Can you work these out from the model? Positions are in its coordinate system, mm. A direction names the side the tool comes from. Give positions to 0.01 mm unless a question says otherwise; leave off trailing zeros. Loops run counter-clockwise (first coordinate to the right, second up) from the corner with the lowest first, then second, coordinate; pieces in that order, holes last. Notation, with made-up numbers: (32.25, 85.25) -> (90.25, 85.25) arc R11 ccw to (90.25, 103.25) -> close; hole circle Ø7 at (34, -32). An arc over 180 degrees is marked (long way). Return JSON: item names as keys, results as strings. Group by question number.
Q1. Will these pins go through, and if not, where does the flat tip stop? pin 1 (12 mm diameter, centred on x = 30.5, y = 23, fed in from -Z); pin 2 (8 mm diameter, centred on y = 22.5, z = -41.5, fed in from -X); pin 3 (3 mm diameter, centred on y = 55, z = -5, fed in from -X) (1 decimal); pin 4 (2 mm diameter, centred on y = 52, z = -27.5, fed in from +X).
Q2. Which directions (+Z, -Z, +X, -X, +Y, -Y) give clear straight access to the entire face, cutting with the end or side of a thin tool? Please do faces 1 (the cylindrical face through (28, 38, -28)), 2 (the cylindrical face through (40, 12, -6)), 3 (the flat face through (20, 53, -7)).
Q3. I need wall thicknesses on line 1 along Z through (x, y) = (15.75, 55); line 2 along Y through (x, z) = (67, -55); line 3 along Z through (x, y) = (71, 3). Which ranges of each line are inside material? Lowest first, please. Write a range as [from, to].
Q4. Suppose I cut it at A-A, the plane z = -15.5. Please give me the cut outline in (x, y), and give its area (3 significant figures).
Q5. Suppose I cut it at B-B, the plane y = 9.5. Please give me the cut outline in (x, z), and give its area (3 significant figures).
Q6. Suppose I cut it at C-C, the plane x = 55. Please give me the cut outline in (y, z).
Q7. Thinking about a two-plate mould opening in Z: for faces 4 (the flat face through (60, 7, -53)), 5 (the cylindrical face through (10, 59, -58)), 6 (the flat face through (98, 35, -32.5)), which applies, pulls with the +Z half, pulls with the -Z half, needs draft (parallel to the pull), parting line crosses it, or undercut?
```python
from build123d import *

# Parameters (mm, degrees)
SKETCH_1_W           = 60
SKETCH_1_H           = 60
EXTRUDE_1_DEPTH      = 20
SKETCH_2_R           = 30
EXTRUDE_2_DEPTH      = 40
SKETCH_3_W           = 60
SKETCH_3_H           = 60
EXTRUDE_3_DEPTH      = 12
SKETCH_4_R           = 22
EXTRUDE_4_DEPTH      = 10
SKETCH_5_R           = 7
EXTRUDE_5_DEPTH      = 22
SKETCH_6_R           = 2.5
CUT_EXTRUDE_1_DEPTH  = 135.223693885
SKETCH_7_R           = 25
CUT_EXTRUDE_2_DEPTH  = 5
SKETCH_8_R           = 7
CUT_EXTRUDE_3_DEPTH  = 25
CUT_EXTRUDE_START    = -15
CUT_EXTRUDE_5_DEPTH  = 15
FILLET_1_R           = 2.5
SKETCH_11_R          = 8
EXTRUDE_6_DEPTH      = 2
M5X0_751_D           = 4.2
M5X0_751_DEPTH       = 14
M5X0_751_CSINK_D     = 6
M5X0_751_CSINK_ANGLE = 90
M5X0_751_TIP         = 1.2618073
FILLET_2_R           = 5
SKETCH_15_W          = 5
SKETCH_15_H          = 2.461651585
CUT_EXTRUDE_6_DEPTH  = 24
FILLET_3_R           = 2.5


with BuildPart() as part:
    # Эскиз1 → Бобышка-Вытянуть1 (new body)
    with BuildSketch(Plane(origin=(0, 0, 0), x_dir=(0, 0, -1), z_dir=(1, 0, 0))):
        with Locations((30, 30)):
            Rectangle(SKETCH_1_W, SKETCH_1_H)
    extrude(amount=EXTRUDE_1_DEPTH)

    # Эскиз2 → Бобышка-Вытянуть2 (add)
    with BuildSketch(Plane(origin=(20, 0, 0), x_dir=(0, 0, -1), z_dir=(1, 0, 0))):
        with Locations((30, 30)):
            Circle(SKETCH_2_R)
    extrude(amount=EXTRUDE_2_DEPTH)

    # Эскиз3 → Бобышка-Вытянуть3 (add)
    with BuildSketch(Plane(origin=(60, 0, 0), x_dir=(0, 0, -1), z_dir=(1, 0, 0))):
        with Locations((30, 30)):
            Rectangle(SKETCH_3_W, SKETCH_3_H)
    extrude(amount=EXTRUDE_3_DEPTH)

    # Эскиз4 → Бобышка-Вытянуть4 (add)
    with BuildSketch(Plane(origin=(72, 0, 0), x_dir=(0, 0, -1), z_dir=(1, 0, 0))):
        with Locations((30, 30)):
            Circle(SKETCH_4_R)
    extrude(amount=EXTRUDE_4_DEPTH)

    # Эскиз5 → Бобышка-Вытянуть5 (add)
    with BuildSketch(Plane(origin=(82, 0, 0), x_dir=(0, 0, -1), z_dir=(1, 0, 0))):
        with Locations((30, 30)):
            Circle(SKETCH_5_R)
    extrude(amount=EXTRUDE_5_DEPTH)

    # Эскиз6 → Вырез-Вытянуть1 (cut, through all)
    with BuildSketch(Plane.ZY):
        with Locations(Location((-55, 55, 0), (0, 0, 180))):
            Circle(SKETCH_6_R)
        with Locations(Location((-5, 55, 0), (0, 0, 180))):
            Circle(SKETCH_6_R)
        with Locations(Location((-5, 5, 0), (0, 0, 180))):
            Circle(SKETCH_6_R)
        with Locations(Location((-55, 5, 0), (0, 0, 180))):
            Circle(SKETCH_6_R)
    extrude(amount=-CUT_EXTRUDE_1_DEPTH, mode=Mode.SUBTRACT)

    # Эскиз7 → Вырез-Вытянуть2 (cut)
    with BuildSketch(Plane.ZY):
        with Locations((-30, 30)):
            Circle(SKETCH_7_R)
    extrude(amount=-CUT_EXTRUDE_2_DEPTH, mode=Mode.SUBTRACT)

    # Эскиз8 → Вырез-Вытянуть3 (cut)
    with BuildSketch(Plane.ZY.offset(-5)):
        with Locations(Location((-30, 30, 0), (0, 0, 180))):
            Circle(SKETCH_8_R)
    extrude(amount=-CUT_EXTRUDE_3_DEPTH, mode=Mode.SUBTRACT)

    # Эскиз10 → Вырез-Вытянуть5 (cut)
    with BuildSketch(Plane(origin=(104, 0, 0), x_dir=(0, 0, -1), z_dir=(1, 0, 0)).offset(CUT_EXTRUDE_START)):
        with BuildLine():
            Line((27.5, 34), (32.5, 34))
            Line((32.5, 34), (32.5, 36.538348415))
            ThreePointArc((32.5, 36.538348415), (30, 37), (27.5, 36.538348415))
            Line((27.5, 36.538348415), (27.5, 34))
        make_face()
    extrude(amount=CUT_EXTRUDE_5_DEPTH, mode=Mode.SUBTRACT)

    # Скругление1
    fillet_1_edges = [part.edges().sort_by_distance(p)[0] for p in [
        (89, 35.269174208, -27.5),
        (89, 35.269174208, -32.5),
    ]]
    fillet(fillet_1_edges, radius=FILLET_1_R - 0.0001)  # a hair under: the kernel refuses the full size

    # Эскиз11 → Бобышка-Вытянуть6 (add)
    with BuildSketch(Plane(origin=(82, 0, 0), x_dir=(0, 0, -1), z_dir=(1, 0, 0))):
        with Locations((30, 30)):
            Circle(SKETCH_11_R)
    extrude(amount=EXTRUDE_6_DEPTH)

    # Отверстие обработанное метчиком M5x0.751
    with Locations(Plane(origin=(104, 0, 0), x_dir=(0, 0, -1), z_dir=(1, 0, 0))):
        with Locations((30, 30)):
            CounterSinkHole(M5X0_751_D / 2, M5X0_751_CSINK_D / 2, depth=M5X0_751_DEPTH, counter_sink_angle=M5X0_751_CSINK_ANGLE)
            with Locations((0, 0, -(M5X0_751_DEPTH + M5X0_751_TIP / 2))):  # 118° drill point
                Cone(0, M5X0_751_D / 2, M5X0_751_TIP, mode=Mode.SUBTRACT)

    # Скругление2
    fillet_2_edges = [part.edges().sort_by_distance(p)[0] for p in [
        (66, 60, 0),
        (66, 0, 0),
        (66, 0, -60),
        (66, 60, -60),
        (10, 60, 0),
        (10, 60, -60),
        (10, 0, -60),
        (10, 0, 0),
    ]]
    fillet(fillet_2_edges, radius=FILLET_2_R)

    # Эскиз15 → Вырез-Вытянуть6 (cut)
    with BuildSketch(Plane.ZY.offset(-5)):
        with Locations((-30, 37.769174208)):
            Rectangle(SKETCH_15_W, SKETCH_15_H)
    extrude(amount=-CUT_EXTRUDE_6_DEPTH, mode=Mode.SUBTRACT)

    # Скругление3
    fillet_3_edges = [part.edges().sort_by_distance(p)[0] for p in [
        (29, 37.769174208, -32.5),
        (29, 37.769174208, -27.5),
    ]]
    fillet(fillet_3_edges, radius=FILLET_3_R - 0.0001)  # a hair under: the kernel refuses the full size


solid = part.part
```
Ans:
{
 "1": {"pin 1": "stops at z = -59.98", "pin 2": "stops at x = 5", "pin 3": "passes through", "pin 4": "stops at x = 82"},
 "2": {"face 1": "-X", "face 2": "none", "face 3": "+Z, +Y"},
 "3": {"line 1": "z = [-60, -57.5], [-52.5, -7.5], [-2.5, 0]", "line 2": "y = [0, 2.5], [7.5, 52.5], [57.5, 60]", "line 3": "z = [-59.58, -56.5], [-53.5, -6.5], [-3.5, -0.42]"},
 "4": {"outline": "(0, 0) -> (20, 0) -> (20, 3.74) -> (60, 3.74) -> (60, 0) -> (72, 0) -> (72, 13.45) -> (82, 13.45) -> (82, 46.55) -> (72, 46.55) -> (72, 60) -> (60, 60) -> (60, 56.26) -> (20, 56.26) -> (20, 60) -> (0, 60) -> (0, 50.37) -> (5, 50.37) -> (5, 9.63) -> (0, 9.63) -> close", "area": "4,150 mm^2"},
 "5": {"outline": "(0, -60) -> (20, -60) -> (20, -51.9) -> (60, -51.9) -> (60, -60) -> (72, -60) -> (72, -37.98) -> (82, -37.98) -> (82, -22.02) -> (72, -22.02) -> (72, 0) -> (60, 0) -> (60, -8.1) -> (20, -8.1) -> (20, 0) -> (0, 0) -> (0, -15.69) -> (5, -15.69) -> (5, -44.31) -> (0, -44.31) -> close", "area": "3,690 mm^2"},
 "6": {"outline": "circle Ø60 at (30, -30)"},
 "7": {"face 4": "needs draft", "face 5": "pulls with the -Z half", "face 6": "undercut"}
}
